Could you check a few things on this model? Use its own coordinates, in mm. A direction names the side the tool comes from. Give positions to 0.01 mm unless a question says otherwise; leave off trailing zeros. Order: outer loops, then holes, each group sorted by start corner. A loop starts at its lowest first (then second) coordinate and runs counter-clockwise, first axis right, second up. Notation, with made-up numbers: M -4,46 L 20,46 A19 cw 20,72 Z; hole C 78.25,89 d6. An arc over 180 degrees is marked long. Answer in a Markdown table with one row per item. Add a question column.
```python
from build123d import *

# Parameters (mm, degrees)
SKETCH_W        = 18.4
SKETCH_H        = 11
PAD_DEPTH       = 8
SKETCH002_R     = 2.6
POCKET_DEPTH    = 10
SKETCH003_W     = 16
SKETCH003_H     = 9.8
POCKET001_DEPTH = 6.8
SKETCH004_W     = 10.8
SKETCH004_H     = 3
POCKET002_DEPTH = 5
SKETCH005_W     = 18.4
SKETCH005_H     = 3
PAD001_DEPTH    = 1.2
SKETCH006_W     = 18.4
SKETCH006_H     = 8
PAD002_DEPTH    = 1.2
FILLET_R        = 1


with BuildPart() as part:
    # Sketch → Pad (new body)
    with BuildSketch(Plane.XY):
        Rectangle(SKETCH_W, SKETCH_H)
    extrude(amount=PAD_DEPTH)

    # Sketch002 (on Face3 of Pad) → Pocket (cut)
    with BuildSketch(Plane(origin=(0, 5.5, 0), x_dir=(-1, 0, 0), z_dir=(0, 1, 0))):
        with Locations((-5.4, 4.8)):
            Circle(SKETCH002_R)
        with Locations((0, 4.8)):
            Circle(SKETCH002_R)
        with Locations((5.4, 4.8)):
            Circle(SKETCH002_R)
    extrude(amount=-POCKET_DEPTH, mode=Mode.SUBTRACT)

    # Sketch003 (on Face5 of Pocket) → Pocket001 (cut)
    with BuildSketch(Plane.XY.offset(8)):
        with Locations((0, -0.6)):
            Rectangle(SKETCH003_W, SKETCH003_H)
    extrude(amount=-POCKET001_DEPTH, mode=Mode.SUBTRACT)

    # Sketch004 (on Face9 of Pocket001) → Pocket002 (cut)
    with BuildSketch(Plane(origin=(0, 5.5, 0), x_dir=(-1, 0, 0), z_dir=(0, 1, 0))):
        with Locations((0, 4.8)):
            Rectangle(SKETCH004_W, SKETCH004_H)
    extrude(amount=-POCKET002_DEPTH, mode=Mode.SUBTRACT)

    # Sketch005 (on Face1 of Pocket002) → Pad001 (join)
    with BuildSketch(Plane.XZ.offset(5.5)):
        with Locations((0, 1.5)):
            Rectangle(SKETCH005_W, SKETCH005_H)
    extrude(amount=PAD001_DEPTH)

    # Sketch006 (on Face4 of Pad001) → Pad002 (join)
    with BuildSketch(Plane.XY.offset(8)):
        with Locations((0, 1.5)):
            Rectangle(SKETCH006_W, SKETCH006_H)
    extrude(amount=PAD002_DEPTH)

    # Fillet
    fillet_edges = [part.edges().sort_by_distance(p)[0] for p in [
        (0, 5.5, 9.2),
        (-9.2, 5.5, 4.6),
        (0, 5.5, 0),
        (9.2, 5.5, 4.6),
        (9.2, 1.5, 9.2),
        (-9.2, 1.5, 9.2),
        (-9.2, -0.6, 0),
        (9.2, -0.6, 0),
    ]]
    fillet(fillet_edges, radius=FILLET_R)


solid = part.part
```
1. Thinking about a two-plate mould opening in Y: for faces 4 (the flat face through (0, 4.3, 2)), 5 (the flat face through (-9, -5.5, 5)), 6 (the flat face through (-3, 5, 6.3)), which applies, pulls with the +Y half, pulls with the -Y half, needs draft (parallel to the pull), parting line crosses it, or undercut?
2. Will these pins go through, and if not, where does the flat tip stop? P1, Ø1.5, axis at x = 5, z = 5.5, coming from the -Y side; P2, Ø2, axis at x = -4, y = -4, coming from the +Z side; P3, Ø0.6, axis at x = -8.5, z = 5.5, coming from the -Y side; P4, Ø1, axis at x = 8.5, y = -4, coming from the +Z side.
3. If I drill on line 1 along X through (y, z) = (-5.25, 7); line 2 along Y through (x, z) = (2.5, 1.5); line 3 along Z through (x, y) = (6.75, 2), over which ranges is the centre line in solid material (lowest first)? Write a range as [from, to].
4. Suppose I cut it at B-B on y = -3.75. List the corners of the cut face in (x, z) for me.
5. Suppose I cut it at C-C on z = 1.75. List the corners of the cut face in (x, y) for me.
6. For faces 1 (the cylindrical face through (0, 4.9, 7.4)), 2 (the flat face through (-9, -4, 8)), 3 (the flat face through (0, -5.5, 2)), which set-ups out of +Z, -Z, +X, -X, +Y, -Y let a thin tool reach every point of the face, with its end or its side?
7. Suppose I cut it at D-D on y = 4.75. List the corners of the cut face in (x, z) for me.
8. Suppose I cut it at A-A on x = -5.4. List the corners of the cut face in (y, z) for me.
Findings below:
| question | item | result |
|---|---|---|
| 1 | face 4 | undercut |
| 1 | face 5 | pulls with the -Y half |
| 1 | face 6 | needs draft |
| 2 | P1 | through |
| 2 | P2 | z = 1.2 |
| 2 | P3 | y = -5.5 |
| 2 | P4 | z = 8 |
| 3 | line 1 | [-9.2, -8], [8, 9.2] |
| 3 | line 2 | [-6.7, -5.5], [4.3, 5.5] |
| 3 | line 3 | [0, 1.2], [8, 9.2] |
| 4 | outline | M -9.2,1 A1 ccw -8.2,0 L 8.2,0 A1 ccw 9.2,1 L 9.2,8 L 8,8 L 8,1.2 L -8,1.2 L -8,8 L -9.2,8 Z |
| 5 | outline | M -9.2,-6.7 L 9.2,-6.7 L 9.2,4.5 A1 ccw 8.2,5.5 L -8.2,5.5 A1 ccw -9.2,4.5 Z; hole M -8,-5.5 L 8,-5.5 L 8,4.3 L -8,4.3 Z |
| 6 | face 1 | +Y, -Y |
| 6 | face 2 | +Z, +X, -X, -Y |
| 6 | face 3 | +Z |
| 7 | outline | M -9.17,1 A0.97 ccw -8.2,0.03 L 8.2,0.03 A0.97 ccw 9.17,1 L 9.17,8.2 A0.97 ccw 8.2,9.17 L -8.2,9.17 A0.97 ccw -9.17,8.2 Z; hole M -3.28,3.3 L -2.12,3.3 A2.6 ccw 2.12,3.3 L 3.28,3.3 A2.6 ccw long 3.28,6.3 L 2.12,6.3 A2.6 ccw -2.12,6.3 L -3.28,6.3 A2.6 ccw long Z |
| 8 | outline | M -6.7,0 L 4.5,0 A1 ccw 5.5,1 L 5.5,2.2 L 4.3,2.2 L 4.3,1.2 L -5.5,1.2 L -5.5,3 L -6.7,3 Z; M -2.5,8 L 4.3,8 L 4.3,7.4 L 5.5,7.4 L 5.5,8.2 A1 ccw 4.5,9.2 L -2.5,9.2 Z |
